Source: CAD feature listing. Evaluate the final solid. Frame: model axes, mm. Face numbers are marked on the shaded views. A direction names the side the tool comes from. Give positions to 0.01 mm unless a question says otherwise; leave off trailing zeros. Write each loop counter-clockwise with the first axis right and the second up, starting at its lowest first coordinate (ties: lowest second). Pieces come first, ordered by that corner, then holes. Notation, with made-up numbers: M -32,-4.75 L 27,-4.75 A16 cw 27,26.25 Z; hole C 12.25,89 d6. An arc over 180 degrees is marked long. Answer as a JSON object with one key per item and string values. Group by question number.
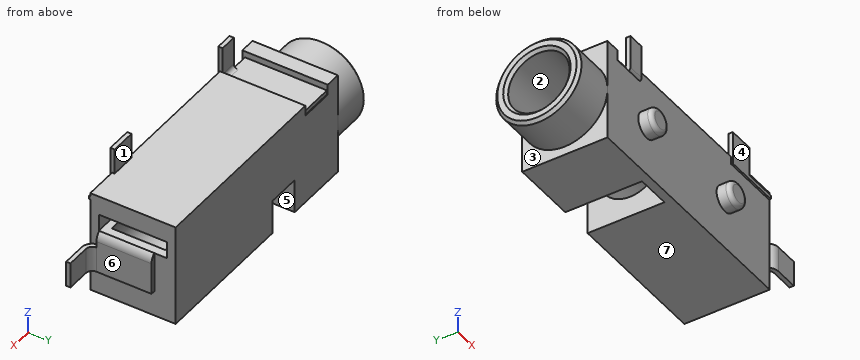
```python
from build123d import *

# Parameters (mm, degrees)
SKETCH1_W            = 0.625
SKETCH1_H            = 1.5
REVOLVE1_ANGLE       = 90
BOSS_EXTRUDE1_DEPTH  = 4.475
SKETCH3_W            = 4.5
SKETCH3_H            = 4.475
BOSS_EXTRUDE2_DEPTH  = 12.6
SKETCH4_W            = 12.6
SKETCH4_H            = 4.5
BOSS_EXTRUDE3_DEPTH  = 0.525
SKETCH5_W            = 1.5
SKETCH5_H            = 5.1
BOSS_EXTRUDE4_DEPTH  = 1.375
SKETCH6_W            = 1.75
SKETCH6_H            = 1.5
CUT_EXTRUDE1_DEPTH   = 4.475
SKETCH7_W            = 1.75
SKETCH7_H            = 1.5
CUT_EXTRUDE2_DEPTH   = 0.375
CUT_EXTRUDE3_START   = -1.25
CUT_EXTRUDE3_DEPTH   = 1.25
SKETCH9_W            = 12.6
SKETCH9_H            = 5
BOSS_EXTRUDE5_DEPTH  = 1.5
BOSS_EXTRUDE6_START  = 1.9
BOSS_EXTRUDE6_DEPTH  = 1
SKETCH11_W           = 5.625
SKETCH11_H           = 5
BOSS_EXTRUDE7_DEPTH  = 1.9
SKETCH12_W           = 0.9
SKETCH12_H           = 5
BOSS_EXTRUDE8_DEPTH  = 0.375
CUT_EXTRUDE4_REACH   = 19.458
SKETCH14_W           = 1
SKETCH14_H           = 0.25
SKETCH15_W           = 1
SKETCH15_H           = 0.375
CUT_EXTRUDE5_DEPTH   = 4.85
SKETCH16_W           = 1
SKETCH16_H           = 0.25
BOSS_EXTRUDE9_DEPTH  = 1.5
BOSS_EXTRUDE10_REACH = 19.847
SKETCH18_W           = 1.5
SKETCH18_H           = 0.25
BOSS_EXTRUDE11_DEPTH = 1.5
SKETCH19_W           = 1
SKETCH19_H           = 4
CUT_EXTRUDE6_DEPTH   = 2
CUT_EXTRUDE7_REACH   = 20.059
SKETCH21_W           = 2
SKETCH21_H           = 0.05
SKETCH22_W           = 2
SKETCH22_H           = 4.5
CUT_EXTRUDE8_DEPTH   = 2
SKETCH23_W           = 2.5
SKETCH23_H           = 2.5
SKETCH24_W           = 0.75
SKETCH24_H           = 0.8
SKETCH25_W           = 0.75
SKETCH25_H           = 0.8
HOLE1_D              = 3.6
HOLE1_DEPTH          = 16.5
CHAMFER1_SIZE        = 0.175
FILLET1_R            = 0.25
FILLET2_R            = 0.375


# Read off the part's stored shape, not the designer's step: Boss-Extrude6
with BuildPart() as part:
    # Sketch1 → Revolve1 (revolve)
    with BuildSketch(Plane(origin=(0, 0.525, 0), x_dir=(1, 0, 0), z_dir=(0, 1, 0))):
        with Locations((14.8125, 0.75)):
            Rectangle(SKETCH1_W, SKETCH1_H)
    revolve(axis=Axis((15.125, 0.525, 0), (0, 0, 1)), revolution_arc=REVOLVE1_ANGLE)

    # Sketch2 → Boss-Extrude1 (add)
    with BuildSketch(Plane(origin=(0, 0.525, 0), x_dir=(-1, 0, 0), z_dir=(0, 1, 0))):
        with BuildLine():
            Line((-14.5, -1.5), (-15.125, -1.5))
            Line((-15.125, -1.5), (-15.125, 0))
            Line((-15.125, 0), (-14.75, 0))
            Line((-14.75, 0), (-14.75, 0.375))
            ThreePointArc((-14.75, 0.375), (-14.684016994, 0.654508497), (-14.5, 0.875))
            Line((-14.5, 0.875), (-14.5, -1.5))
        make_face()
    extrude(amount=BOSS_EXTRUDE1_DEPTH)

    # Sketch3 → Boss-Extrude2 (add)
    with BuildSketch(Plane.ZY.offset(-14.5)):
        with Locations((0.75, 2.7625)):
            Rectangle(SKETCH3_W, SKETCH3_H)
    extrude(amount=BOSS_EXTRUDE2_DEPTH)

    # Sketch4 → Boss-Extrude3 (add)
    with BuildSketch(Plane.XZ.offset(-0.525)):
        with Locations((8.2, 0.75)):
            Rectangle(SKETCH4_W, SKETCH4_H)
    extrude(amount=BOSS_EXTRUDE3_DEPTH)

    # Sketch5 → Boss-Extrude4 (add)
    with BuildSketch(Plane(origin=(15.125, 0, 0), x_dir=(0, 0, -1), z_dir=(1, 0, 0))):
        with Locations((0.75, 2.45)):
            Rectangle(SKETCH5_W, SKETCH5_H)
    extrude(amount=BOSS_EXTRUDE4_DEPTH)

    # Sketch6 → Cut-Extrude1 (cut)
    with BuildSketch(Plane(origin=(0, 5, 0), x_dir=(-1, 0, 0), z_dir=(0, 1, 0))):
        with Locations((-15.625, -0.75)):
            Rectangle(SKETCH6_W, SKETCH6_H)
    extrude(amount=-CUT_EXTRUDE1_DEPTH, mode=Mode.SUBTRACT)

    # Sketch7 → Cut-Extrude2 (cut)
    with BuildSketch(Plane(origin=(0, 0.525, 0), x_dir=(-1, 0, 0), z_dir=(0, 1, 0))):
        with Locations((-15.625, -0.75)):
            Rectangle(SKETCH7_W, SKETCH7_H)
    extrude(amount=-CUT_EXTRUDE2_DEPTH, mode=Mode.SUBTRACT)

    # Sketch8 → Cut-Extrude3 (cut)
    with BuildSketch(Plane(origin=(0, 5, 0), x_dir=(-1, 0, 0), z_dir=(0, 1, 0)).offset(CUT_EXTRUDE3_START)):
        with BuildLine():
            Line((-14.75, -1.5), (-14.5, -1.5))
            Line((-14.5, -1.5), (-14.5, 0.875))
            ThreePointArc((-14.5, 0.875), (-14.684016994, 0.654508497), (-14.75, 0.375))
            Line((-14.75, 0.375), (-14.75, -1.5))
        make_face()
    extrude(amount=CUT_EXTRUDE3_DEPTH, mode=Mode.SUBTRACT)

    # Sketch9 → Boss-Extrude5 (add)
    with BuildSketch(Plane(origin=(0, 0, -1.5), x_dir=(-1, 0, 0), z_dir=(0, 0, -1))):
        with Locations((-8.2, 2.5)):
            Rectangle(SKETCH9_W, SKETCH9_H)
    extrude(amount=BOSS_EXTRUDE5_DEPTH)

    # Boss-Extrude6 outline → Boss-Extrude6 (add)
    with BuildSketch(Plane.YZ.offset(BOSS_EXTRUDE6_START)):
        with BuildLine():
            Line((0, 3), (-0.1, 3))
            Line((-0.1, 3), (-0.1, 2.548205081))
            ThreePointArc((-0.1, 2.548205081), (-0.073205081, 2.448205081), (0, 2.375))
            Line((0, 2.375), (0, 3))
        make_face()
    extrude(amount=BOSS_EXTRUDE6_DEPTH)

    # Sketch11 → Boss-Extrude7 (add)
    with BuildSketch(Plane.ZY.offset(-1.9)):
        with Locations((-0.1875, 2.5)):
            Rectangle(SKETCH11_W, SKETCH11_H)
    extrude(amount=BOSS_EXTRUDE7_DEPTH)

    # Sketch12 → Boss-Extrude8 (add)
    with BuildSketch(Plane.XY.offset(2.625)):
        with Locations((0.45, 2.5)):
            Rectangle(SKETCH12_W, SKETCH12_H)
    extrude(amount=BOSS_EXTRUDE8_DEPTH)

    # Sketch14 → Cut-Extrude4 (cut, up to next)
    with BuildSketch(Plane(origin=(0, 0.15, 0), x_dir=(1, 0, 0), z_dir=(0, 1, 0)), mode=Mode.PRIVATE) as cut_extrude4_sk1:
        with Locations((1.4, -2.5)):
            Rectangle(SKETCH14_W, SKETCH14_H)
    cut_extrude4_tool1 = extrude(cut_extrude4_sk1.sketch, amount=-CUT_EXTRUDE4_REACH, mode=Mode.PRIVATE) & part.part
    add(cut_extrude4_tool1.solids().sort_by_distance((1.4, 0.15, 2.5))[0], mode=Mode.SUBTRACT)

    # Sketch15 → Cut-Extrude5 (cut)
    with BuildSketch(Plane(origin=(0, 5, 0), x_dir=(-1, 0, 0), z_dir=(0, 1, 0))):
        with Locations((-2.4, 2.8125)):
            Rectangle(SKETCH15_W, SKETCH15_H)
    extrude(amount=-CUT_EXTRUDE5_DEPTH, mode=Mode.SUBTRACT)

    # Sketch16 → Boss-Extrude9 (add)
    with BuildSketch(Plane.XY.offset(3)):
        with Locations((2.4, 0.025)):
            Rectangle(SKETCH16_W, SKETCH16_H)
    extrude(amount=BOSS_EXTRUDE9_DEPTH)

    # Sketch17 → Boss-Extrude10 (add, up to next)
    with BuildSketch(Plane.XZ.offset(0.1), mode=Mode.PRIVATE) as boss_extrude10_sk1:
        Polygon((12.55, 2.775), (12.55, 3), (11.05, 3), (11.05, 2.548205081), (14.45, 2.548205081), (14.45, 2.775), align=None)
    boss_extrude10_tool1 = extrude(boss_extrude10_sk1.sketch, amount=-BOSS_EXTRUDE10_REACH, mode=Mode.PRIVATE) - part.part
    add(boss_extrude10_tool1.solids().sort_by_distance((12.460785, -0.1, 2.730374))[0])

    # Sketch18 → Boss-Extrude11 (add)
    with BuildSketch(Plane.XY.offset(3)):
        with Locations((11.8, 0.025)):
            Rectangle(SKETCH18_W, SKETCH18_H)
    extrude(amount=BOSS_EXTRUDE11_DEPTH)

    # Sketch19 → Cut-Extrude6 (cut)
    with BuildSketch(Plane(origin=(14.5, 0, 0), x_dir=(0, 0, -1), z_dir=(1, 0, 0))):
        with Locations((-1.375, 2.5)):
            Rectangle(SKETCH19_W, SKETCH19_H)
    extrude(amount=-CUT_EXTRUDE6_DEPTH, mode=Mode.SUBTRACT)

    # Sketch21 → Cut-Extrude7 (cut, up to next)
    with BuildSketch(Plane(origin=(0, 0, 2.375), x_dir=(-1, 0, 0), z_dir=(0, 0, -1)), mode=Mode.PRIVATE) as cut_extrude7_sk1:
        with Locations((-1.9, 4.975)):
            Rectangle(SKETCH21_W, SKETCH21_H)
    cut_extrude7_tool1 = extrude(cut_extrude7_sk1.sketch, amount=-CUT_EXTRUDE7_REACH, mode=Mode.PRIVATE) & part.part
    add(cut_extrude7_tool1.solids().sort_by_distance((1.9, 4.975, 2.375))[0], mode=Mode.SUBTRACT)

    # Sketch22 → Cut-Extrude8 (cut)
    with BuildSketch(Plane(origin=(0, 0, -3), x_dir=(-1, 0, 0), z_dir=(0, 0, -1))):
        with Locations((-4.85, 2.75)):
            Rectangle(SKETCH22_W, SKETCH22_H)
    extrude(amount=-CUT_EXTRUDE8_DEPTH, mode=Mode.SUBTRACT)

    # Sketch23 → Revolve2 (revolve)
    with BuildSketch(Plane.XY, mode=Mode.PRIVATE) as revolve2_sk:
        with Locations((-1.25, 3.75)):
            Rectangle(SKETCH23_W, SKETCH23_H)
    revolve(revolve2_sk.sketch.rotate(Axis((-2.5, 2.5, 0), (1, 0, 0)), 270), axis=Axis((-2.5, 2.5, 0), (1, 0, 0)))

    # Sketch24 → Revolve3 (revolve)
    with BuildSketch(Plane.XY, mode=Mode.PRIVATE) as revolve3_sk:
        with Locations((3.875, -0.4)):
            Rectangle(SKETCH24_W, SKETCH24_H)
    revolve(revolve3_sk.sketch.rotate(Axis((3.5, 0, 0), (0, -1, 0)), 270), axis=Axis((3.5, 0, 0), (0, -1, 0)))

    # Sketch25 → Revolve4 (revolve)
    with BuildSketch(Plane.XY, mode=Mode.PRIVATE) as revolve4_sk:
        with Locations((10.875, -0.4)):
            Rectangle(SKETCH25_W, SKETCH25_H)
    revolve(revolve4_sk.sketch.rotate(Axis((10.5, 0, 0), (0, -1, 0)), 270), axis=Axis((10.5, 0, 0), (0, -1, 0)))

    # Hole1
    with Locations(Plane.ZY.offset(2.5)):
        with Locations((0, 2.5)):
            Hole(HOLE1_D / 2, depth=HOLE1_DEPTH)

    # Chamfer1
    chamfer1_edges = [part.edges().sort_by_distance(p)[0] for p in [
        (-2.5, 2.5, 2.5),
        (-2.5, 2.5, 1.8),
    ]]
    chamfer(chamfer1_edges, length=CHAMFER1_SIZE)

    # Fillet1
    fillet1_edges = [part.edges().sort_by_distance(p)[0] for p in [
        (2.4, 0.15, 2.625),
        (3.5, -0.8, 0.75),
        (10.5, -0.8, 0.75),
    ]]
    fillet(fillet1_edges, radius=FILLET1_R)

    # Fillet2
    fillet2_edges = [part.edges().sort_by_distance(p)[0] for p in [
        (14.75, 0.15, -0.75),
    ]]
    fillet(fillet2_edges, radius=FILLET2_R)


solid = part.part
```
(1) Section D-D, the plane x = 15.5. Return loops of the section in (y, z).
(2) Section A-A, the plane y = 2.5. State how many separate pieces and enclosed holes the cut face has, plus the area to 3 significant figures.
(3) Contact query for flat-ended pins moving along their axis: pin 1 Ø1.8 at (x, z) = (5, 1.5) entering from -Y; pin 2 Ø0.7 at (x, y) = (0.5, 2) entering from +Z; pin 3 Ø0.7 at (x, z) = (15.5, -0.5) entering from -Y. Output: stop coordinate, or through.
(4) Section B-B, the plane x = 10.5. Return loops of the section in (y, z), plus the area to 3 significant figures.
(5) Section C-C, the plane y = -0.3. Return loops of the section in (x, z), plus the area to 3 significant figures.
(6) Access query for the marked faces 1, 2, 3 and 4. Directions: +Z, -Z, +X, -X, +Y, -Y. A direction counts if a zero-diameter tool reaches every point of the face in a straight line with its end or side. Return the directions, or none.
(7) Pull-direction query (X, two-part tool) for the marked faces 5, 6 and 7; classes: pulls with the +X half, pulls with the -X half, needs draft (parallel to the pull), parting line crosses it, or undercut.
(8) Ray query, L1, parallel to Z at x = 10.75, y = 2.5; L2, parallel to Y at x = 10.75, z = 0; L3, parallel to X at y = 4.4, z = -2. Return the intervals inside material, ascending. Write a range as [from, to].
Reported:
{
 "1": {"outline": "M -0.1,-1.5 L 0.15,-1.5 L 0.15,0 L -0.1,0 Z"},
 "2": {"separate pieces": "3", "enclosed holes": "0", "area": "36.8 mm2"},
 "3": {"pin 1": "stops at y = 0", "pin 2": "stops at z = 3", "pin 3": "stops at y = -0.1"},
 "4": {"outline": "M -0.8,-0.5 A0.25 ccw -0.55,-0.75 L 0,-0.75 L 0,-3 L 5,-3 L 5,3 L 0,3 L 0,0.75 L -0.55,0.75 A0.25 ccw -0.8,0.5 Z; hole C 2.5,0 d3.6", "area": "21.0 mm2"},
 "5": {"outline": "C 3.5,0 d1.5; C 10.5,0 d1.5", "area": "3.53 mm2"},
 "6": {"face 1": "+Z, +X, -X, +Y", "face 2": "-X", "face 3": "-Z, -X", "face 4": "+Z, +X, -X, -Y"},
 "7": {"face 5": "undercut", "face 6": "pulls with the +X half", "face 7": "needs draft"},
 "8": {"L1": "z = [-3, -1.8], [1.8, 3]", "L2": "y = [-0.8, 0.7], [4.3, 5]", "L3": "x = [0, 3.85], [5.85, 14.5]"}
}
